Can you work these out from the model? Positions are in its coordinate system, mm. A direction names the side the tool comes from. Round coordinates to 2 decimals unless told otherwise and drop trailing zeros. Write each loop counter-clockwise with the first axis right and the second up, starting at its lowest first coordinate (ties: lowest second). Pieces come first, ordered by that corner, then holes. Notation, with made-up numbers: (31, 82.5) -> (39, 82.5) arc R22 ccw to (39, 118.5) -> close; hole circle Ø1 at (-11.75, 56.25). An arc over 180 degrees is marked (long way). Write item = value, one per line. Start each with the question number.
1) For faces 1 (the face through (-18, 32, 22)), 2 (the face through (-5, 0, 22)), 3 (the face through (37.7, -2.27, 21.8)), which set-ups out of +Z, -Z, +X, -X, +Y, -Y let a thin tool reach every point of the face, with its end or its side?
2) If I drill on line 1 (Y direction, x = -15, z = 9); line 2 (Y direction, x = -18.5, z = 15); line 3 (Y direction, x = 13.5, z = 40), over which ranges is the centre line in solid material (lowest first)?
3) Imagine slicing it at C-C, the plane x = -13. Please give me the cut outline in (y, z), then the cut area to 3 significant figures.
4) Imagine slicing it at A-A, the plane y = 15.5. Please give me the cut outline in (x, z).
5) Thinking about a two-plate mould opening in Y: for faces 4 (the face through (-6.006, 30.414, 21.199)), 5 (the face through (-22, 14, 22)), 6 (the face through (-26, 4, 22)), which applies, +Y half, -Y half, draft (parallel to the pull), parting line (faces both ways), or undercut?
6) I'm going to push flat-ended pins straight in: pin 1 (12 mm diameter, centred on x = 41, z = 31, fed in from -Y); pin 2 (1 mm diameter, centred on x = -20.5, z = 21.5, fed in from +Y); pin 3 (12 mm diameter, centred on y = -12, z = 25, fed in from +X). Where does each tip first touch, or does it pass through?
7) Imagine slicing it at D-D, the plane y = 34. Please give me the cut outline in (x, z), then the cut area to 3 significant figures.
8) Imagine slicing it at B-B, the plane z = 21.5. Please give me the cut outline in (x, y), then the cut area to 3 significant figures.
from build123d import *

# Parameters (mm, degrees)
SKETCH1_W              = 43
SKETCH1_H              = 32
BOSS_EXTRUDE1_DEPTH    = 29
SKETCH2_W              = 43
SKETCH2_H              = 38
SKETCH2_H_2            = 19
BOSS_EXTRUDE2_DEPTH    = 52
CHAMFER1_SIZE          = 7
SKETCH3_R              = 7
CUT_EXTRUDE1_DEPTH     = 78.440299586
CHAMFER2_SIZE          = 5
SPLIT1_SURFACE_1_BACK  = 108.977
SPLIT1_SURFACE_1_DEPTH = 217.954
CUT_EXTRUDE2_DEPTH     = 52
CUT_EXTRUDE7_DEPTH     = 78.440299586


with BuildPart() as part:
    # Sketch1 → Boss-Extrude1 (new body)
    with BuildSketch(Plane(origin=(0, 0, 0), x_dir=(0, 0, -1), z_dir=(1, 0, 0))):
        with Locations((-21.5, 16)):
            Rectangle(SKETCH1_W, SKETCH1_H)
    extrude(amount=-BOSS_EXTRUDE1_DEPTH)

    # Sketch2 → Boss-Extrude2 (add)
    with BuildSketch(Plane(origin=(0, 0, 0), x_dir=(0, 0, -1), z_dir=(1, 0, 0))):
        with Locations((-21.5, 19)):
            Rectangle(SKETCH2_W, SKETCH2_H)
        with Locations((-21.5, -9.5)):
            Rectangle(SKETCH2_W, SKETCH2_H_2)
    extrude(amount=BOSS_EXTRUDE2_DEPTH)

    # Chamfer1
    chamfer1_edges = [part.edges().sort_by_distance(p)[0] for p in [
        (-29, 0, 21.5),
        (-29, 32, 21.5),
    ]]
    chamfer(chamfer1_edges, length=CHAMFER1_SIZE)

    # Sketch3 → Cut-Extrude1 (cut, through all)
    with BuildSketch(Plane.XY.offset(43)):
        with Locations((-15, 14)):
            Circle(SKETCH3_R)
    extrude(amount=-CUT_EXTRUDE1_DEPTH, mode=Mode.SUBTRACT)

    # Chamfer2
    chamfer2_edges = [part.edges().sort_by_distance(p)[0] for p in [
        (52, 38, 21.5),
    ]]
    chamfer(chamfer2_edges, length=CHAMFER2_SIZE)

    # Split1: cut with a surface, the side behind it stays
    # Split1 surface: a surface, the sketch's curves swept straight by 217.954 mm
    with BuildLine(Plane.XY.offset(-SPLIT1_SURFACE_1_BACK), mode=Mode.PRIVATE) as split1_surface_1_path:
        Line((-15, 32), (3.243084988, 28.783251905))
        ThreePointArc((3.243084988, 28.783251905), (14.574972961, 30.276069151), (23, 38))
    split1_surface_1 = Shell.extrude(split1_surface_1_path.wire(), (0 * SPLIT1_SURFACE_1_DEPTH, 0 * SPLIT1_SURFACE_1_DEPTH, 1 * SPLIT1_SURFACE_1_DEPTH))
    split(bisect_by=split1_surface_1, keep=Keep.BOTTOM)

    # Sketch6 → Cut-Extrude2 (cut)
    with BuildSketch(Plane.XY.offset(43)):
        Polygon((52, -19), (52, 14), (23, -19), align=None)
    extrude(amount=-CUT_EXTRUDE2_DEPTH, mode=Mode.SUBTRACT)

    # Sketch7 → Cut-Extrude7 (cut, through all)
    with BuildSketch(Plane.XY.offset(43)):
        with BuildLine():
            ThreePointArc((17.788067397, -19), (12.527518408, -10.140064923), (10.696969697, 0))
            Line((10.696969697, 0), (0, 0))
            Line((0, 0), (0, -19))
            Line((0, -19), (17.788067397, -19))
        make_face()
    extrude(amount=-CUT_EXTRUDE7_DEPTH, mode=Mode.SUBTRACT)


solid = part.part
Reported:
q1.face_1 = +Z, -Z, -X, +Y
q1.face_2 = +Z, -Z, -X, -Y
q1.face_3 = +Z, -Z, +X, -Y
q2.line_1 = 0 to 7, 21 to 32
q2.line_2 = 0 to 7.94, 20.06 to 32
q2.line_3 = -12.44 to 29.81
q3.outline = (0, 0) -> (7.29, 0) -> (7.29, 43) -> (0, 43) -> close; (20.71, 0) -> (31.65, 0) -> (31.65, 43) -> (20.71, 43) -> close
q3.area = 784 mm²
q4.outline = (-29, 0) -> (-21.84, 0) -> (-21.84, 43) -> (-29, 43) -> close; (-8.16, 0) -> (52, 0) -> (52, 43) -> (-8.16, 43) -> close
q5.face_4 = +Y half
q5.face_5 = undercut
q5.face_6 = -Y half
q6.pin_1 = -5.34
q6.pin_2 = 32
q6.pin_3 = 34.42
q7.outline = (19.92, 0) -> (51, 0) -> (51, 43) -> (19.92, 43) -> close
q7.area = 1,340 mm²
q8.outline = (-29, 7) -> (-22, 0) -> (10.7, 0) arc R29 ccw to (17.79, -19) -> (23, -19) -> (52, 14) -> (52, 33) -> (47, 38) -> (23, 38) arc R19 cw to (3.24, 28.78) -> (-15, 32) -> (-22, 32) -> (-29, 25) -> close; hole circle Ø14 at (-15, 14)
q8.area = 2,760 mm²
